from build123d import *

# Parameters (mm, degrees)
CHAMFER1_SIZE = 0.508


with BuildPart() as part:
    # Sketch2 → Revolve1 (revolve)
    with BuildSketch(Plane.XY, mode=Mode.PRIVATE) as revolve1_sk:
        Polygon((-8.621617421, 5.55625), (-12.7, 5.55625), (-12.7, 4.075), (-8.399999964, 4.075), (-8.399999964, 2.805), (-7.891999964, 2.297), (-7.891999964, 1.905), (-2.748, 1.905), (-0.843, 0), (0, 0), (0, 4.318), (-5.903478608, 4.318), (-6.618382579, 5.55625), (-7.253382579, 5.55625), (-7.62, 4.92125), (-8.255, 4.92125), align=None)
    revolve(revolve1_sk.sketch.rotate(Axis((-12.7, 0, 0), (1, 0, 0)), 180), axis=Axis((-12.7, 0, 0), (1, 0, 0)))

    # Chamfer1
    chamfer1_edges = [part.edges().sort_by_distance(p)[0] for p in [
        (-12.7, 4.075, 0),
    ]]
    chamfer(chamfer1_edges, length=CHAMFER1_SIZE)

    # Mirror1: part across plane


with BuildPart() as part_1:
    add(part.part)
    add(part.part.mirror(Plane(origin=(0, 0, 0), x_dir=(0, 0, 1), z_dir=(1, 0, 0))))


solid = part_1.part
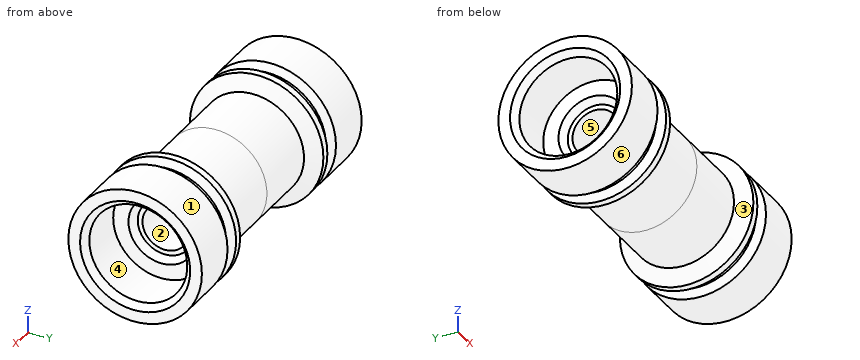
Work out the finished part from the listing and answer in its coordinate system (mm). Face numbers are marked on the shaded views. A direction names the side the tool comes from. Round coordinates to 2 decimals unless told otherwise and drop trailing zeros. Write each loop counter-clockwise with the first axis right and the second up, starting at its lowest first coordinate (ties: lowest second). Pieces come first, ordered by that corner, then holes.
1) A cutting plane is placed at C-C (x = 2.5). Give the vertices of the cut face in (y, z).
2) Given pin 1 Ø6.5 at (y, z) = (0.5, 0.5) entering from -X; pin 2 Ø5 at (y, z) = (1, -2) entering from +X; pin 3 Ø4 at (y, z) = (1.5, 1.5) entering from +X; pin 4 Ø2.5 at (y, z) = (0, 0) entering from -X, each flat-ended and moving along its own axis, determine where each tip first touches the part or whether it passes through.
3) A tool of negligible diameter and unlimited length cuts with its end or side. For the marked faces 3, 4, 5 and 6, from which of +Z, -Z, +X, -X, +Y, -Y can it reach the whole face along a straight path? Write none if from no direction.
4) A cutting plane is placed at B-B (z = 5.25). Give the number of separate pieces and of enclosed holes in the cut face, plus the area to 3 significant figures.
5) The mould has two halves that part along Z. Classify the marked faces 1 and 2: pulls with the +Z half, pulls with the -Z half, needs draft (parallel to the pull), parting line crosses it, or undercut.
6) Straight lines are drawn through the part: line 1 (X direction, y = -4, z = 3); line 2 (Z direction, x = -11.2, y = 0) (3 decimals); line 3 (X direction, y = 2.25, z = -3.25). For each, find the intervals that lie inside material, in ascending order.
Completed:
1. outline: circle Ø8.64 at (0, 0); hole circle Ø3.31 at (0, 0)
2. pin 1: stops at x = -8.4
2. pin 2: stops at x = 12.7
2. pin 3: stops at x = 12.24
2. pin 4: stops at x = -2.09
3. face 3: none
3. face 4: +X
3. face 5: -X
3. face 6: +X, -X
4. separate pieces: 4
4. enclosed holes: 0
4. area: 36.9 mm2
5. face 1: parting line crosses it
5. face 2: undercut
6. line 1: x = -12.7 to -8.3, -7.57 to -6.3, 6.3 to 7.57, 8.3 to 12.7
6. line 2: z = -5.556 to -4.075, 4.075 to 5.556
6. line 3: x = -8.4 to 8.4
